from build123d import *

# Parameters (mm, degrees)
SKETCH1_W           = 168
SKETCH1_H           = 22
BOSS_EXTRUDE1_DEPTH = 17.8
SKETCH8_R           = 2
CUT_EXTRUDE4_DEPTH  = 22
CUT_EXTRUDE2_REACH  = 88.567
SKETCH5_W           = 117
SKETCH5_H           = 6
CUT_EXTRUDE3_DEPTH  = 15.8
BOSS_EXTRUDE2_REACH = 90.164
SKETCH9_W           = 47
SKETCH9_H           = 2


with BuildPart() as part:
    # Sketch1 → Boss-Extrude1 (new body)
    with BuildSketch(Plane(origin=(0, 0, 0), x_dir=(1, 0, 0), z_dir=(0, 1, 0))):
        Rectangle(SKETCH1_W, SKETCH1_H)
    extrude(amount=-BOSS_EXTRUDE1_DEPTH)

    # Sketch8 → Cut-Extrude4 (cut)
    with BuildSketch(Plane.XY.offset(11)):
        with Locations((75.8, -13.35)):
            Circle(SKETCH8_R)
    extrude(amount=-CUT_EXTRUDE4_DEPTH, mode=Mode.SUBTRACT)

    # Cut-Extrude2: up to this face of the body (flat: up to its plane)
    cut_extrude2_end = Plane(part.part.faces().sort_by_distance((0, -17.8, 0))[0])
    # Sketch5 → Cut-Extrude2 (cut, up to the picked face)
    with BuildSketch(Plane(origin=(0, 0, 0), x_dir=(1, 0, 0), z_dir=(0, 1, 0)), mode=Mode.PRIVATE) as cut_extrude2_sk1:
        with Locations((25.5, -8)):
            Rectangle(SKETCH5_W, SKETCH5_H)
    cut_extrude2_tool1 = split(extrude(cut_extrude2_sk1.sketch, amount=-CUT_EXTRUDE2_REACH, mode=Mode.PRIVATE), bisect_by=cut_extrude2_end, keep=Keep.BOTH, mode=Mode.PRIVATE)
    add(cut_extrude2_tool1.solids().sort_by(Axis((25.5, 0, 8), (0, -1, 0)))[0], mode=Mode.SUBTRACT)

    # Sketch6 → Cut-Extrude3 (cut)
    with BuildSketch(Plane.XZ.offset(17.8)):
        Polygon((-82, 9), (-82, -9), (82, -9), (82, 3), (-35, 3), (-35, 9), align=None)
    extrude(amount=-CUT_EXTRUDE3_DEPTH, mode=Mode.SUBTRACT)

    # Boss-Extrude2: up to this face of the body (flat: up to its plane)
    boss_extrude2_end = Plane(part.part.faces().sort_by_distance((-0.369393652, -9.883187228, -9))[0])
    # Sketch9 → Boss-Extrude2 (add, up to the picked face)
    with BuildSketch(Plane(origin=(0, 0, 9), x_dir=(-1, 0, 0), z_dir=(0, 0, -1)), mode=Mode.PRIVATE) as boss_extrude2_sk1:
        with Locations((58.5, -13.3)):
            Rectangle(SKETCH9_W, SKETCH9_H)
    boss_extrude2_tool1 = split(extrude(boss_extrude2_sk1.sketch, amount=BOSS_EXTRUDE2_REACH, mode=Mode.PRIVATE), bisect_by=boss_extrude2_end, keep=Keep.BOTH, mode=Mode.PRIVATE)
    add(boss_extrude2_tool1.solids().sort_by(Axis((-58.5, -13.3, 9), (0, 0, -1)))[0])


solid = part.part
Check sheet for the modelled part. Datum: model origin and axes. Units: mm. A direction names the side the tool comes from. Round coordinates to 2 decimals unless told otherwise and drop trailing zeros. Loops run counter-clockwise (first coordinate to the right, second up) from the corner with the lowest first, then second, coordinate; pieces in that order, holes last.
1. Sectioned sample at A-A on x = -72.5. Record the boundary of the cut face in (y, z), and give its area (3 significant figures).
2. Mould release check, pull along Y, two halves, no side actions. Record for faces 1 (the flat face through (82, -10, -3)), 2 (the flat face through (-1, 0, -3)), 3 (the flat face through (-0.4, -17.8, 3.2)), 4 (the flat face through (-1, -10, -9)): released by +Y, released by -Y, zero draft, split by the parting line, or undercut.
3. Set-up check for faces 5 (the flat face through (-35, -16, 6)), 6 (the flat face through (-84, -9, 0)), 7 (the flat face through (25, -9, 5)), 8 (the flat face through (-35, -7, 6)): record each of +Z, -Z, +X, -X, +Y, -Y from which the full face is reachable in a straight line by a thin tool's end or side.
4. Gauge pin test, flat ends, axial feed: pin 1 Ø4.5 at (x, y) = (11, -8) entering from +Z; pin 2 Ø6.5 at (y, z) = (-12.5, 8.5) entering from +X. Record the tip position at first contact, or that the pin passes through.
5. Sectioned sample at B-B on y = -4. Record the boundary of the cut face in (x, z).
6. Sectioned sample at D-D on x = 55. Record the boundary of the cut face in (y, z), and give its area (3 significant figures).
7. Scan lines: probe 1 along Y at (x, z) = (-67.5, -4.75); probe 2 along Y at (x, z) = (75.8, -9.7); probe 3 along X at (y, z) = (-14, -8.25). Record each from-to range of solid material in increasing order.
8. Sectioned sample at C-C on x = 75.8. Record the boundary of the cut face in (y, z).
Recorded:
1. outline: (-17.8, -11) - (0, -11) - (0, 11) - (-17.8, 11) - (-17.8, 9) - (-14.3, 9) - (-14.3, -9) - (-17.8, -9) - close; hole (-12.3, -9) - (-2, -9) - (-2, 9) - (-12.3, 9) - close
1. area: 143 mm2
2. face 1: zero draft
2. face 2: released by +Y
2. face 3: released by -Y
2. face 4: undercut
3. face 5: -Y
3. face 6: +Z, -Z, -X, +Y, -Y
3. face 7: +Z, +X, +Y, -Y
3. face 8: none
4. pin 1: stops at z = 5
4. pin 2: stops at x = -33
5. outline: (-84, -11) - (84, -11) - (84, 5) - (-33, 5) - (-33, 11) - (-84, 11) - close; hole (-82, -9) - (82, -9) - (82, 3) - (-35, 3) - (-35, 9) - (-82, 9) - close
6. outline: (-17.8, -11) - (0, -11) - (0, 5) - (-17.8, 5) - (-17.8, 3) - (-2, 3) - (-2, -9) - (-17.8, -9) - close
6. area: 95.2 mm2
7. probe 1: y = -14.3 to -12.3, -2 to 0
7. probe 2: y = -17.8 to -15.35, -11.35 to 0
7. probe 3: x = -84 to -35, 82 to 84
8. outline: (-17.8, -11) - (-15.35, -11) - (-15.35, -9) - (-17.8, -9) - close; (-17.8, 3) - (-15.35, 3) - (-15.35, 5) - (-17.8, 5) - close; (-11.35, -11) - (0, -11) - (0, 5) - (-11.35, 5) - (-11.35, 3) - (-2, 3) - (-2, -9) - (-11.35, -9) - close
